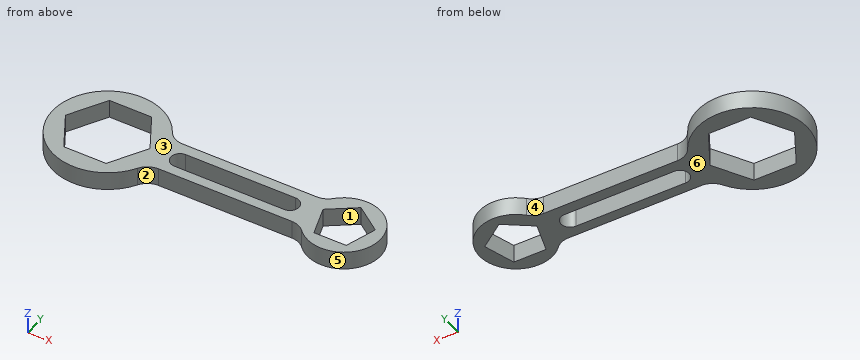
from build123d import *

# Parameters (mm, degrees)
BOSS_EXTRUDE1_DEPTH = 10


with BuildPart() as part:
    # Sketch1 → Boss-Extrude1 (new body)
    with BuildSketch(Plane.XY):
        with BuildLine():
            Line((34.148205858, 10.830267321), (107.410651623, 10.830267321))
            ThreePointArc((107.410651623, 10.830267321), (111.319985045, 11.626077395), (114.607101082, 13.886844881))
            ThreePointArc((114.607101082, 13.886844881), (148.999427872, -0.151277258), (114.398677604, -13.667530292))
            ThreePointArc((114.398677604, -13.667530292), (111.076857226, -11.326938473), (107.098016406, -10.501295438))
            Line((107.098016406, -10.501295438), (34.346715787, -10.501295438))
            ThreePointArc((34.346715787, -10.501295438), (29.409775368, -11.80493877), (25.76003684, -15.375971579))
            ThreePointArc((25.76003684, -15.375971579), (-29.999653993, -0.144084298), (25.611154394, 15.622700491))
            ThreePointArc((25.611154394, 15.622700491), (29.253089327, 12.110299767), (34.148205858, 10.830267321))
        make_face()
        Polygon((11.547005384, 20), (-11.547005384, 20), (-23.094010768, 0), (-11.547005384, -20), (11.547005384, -20), (23.094010768, 0), align=None, mode=Mode.SUBTRACT)
        Polygon((129, 15), (114.734152256, 4.635254916), (120.183221216, -12.135254916), (137.816778784, -12.135254916), (143.265847744, 4.635254916), align=None, mode=Mode.SUBTRACT)
        with BuildLine():
            Line((39.5, 5), (99.5, 5))
            ThreePointArc((99.5, 5), (104.5, 0), (99.5, -5))
            Line((99.5, -5), (39.5, -5))
            ThreePointArc((39.5, -5), (34.5, 0), (39.5, 5))
        make_face(mode=Mode.SUBTRACT)
    extrude(amount=BOSS_EXTRUDE1_DEPTH)


solid = part.part
The model under review builds one solid part; all positions refer to its coordinate system, in mm. Face numbers are marked on the shaded views. A direction names the side the tool comes from. Give positions to 0.01 mm unless a question says otherwise; leave off trailing zeros. Loops run counter-clockwise (first coordinate to the right, second up) from the corner with the lowest first, then second, coordinate; pieces in that order, holes last. Notation, with made-up numbers: (-22, 35.5) -> (24, 35.5) arc R27 ccw to (24, 70.5) -> close; hole circle Ø3 at (36.25, 23). An arc over 180 degrees is marked (long way). Put each result on its own line as item: value. Start each with the question number.
1. We need section A-A on x = 0. State the section outline as (y, z) points.
2. We need section C-C on y = 8. State the section outline as (x, z) points, then the cut area to 3 significant figures.
3. We need section B-B on z = 8. State the section outline as (x, y) points, then the cut area to 3 significant figures.
4. Wall thickness on probe 1 along Y at (x, z) = (76.5, 5.75); probe 2 along X at (y, z) = (-0.5, 9.25); probe 3 along X at (y, z) = (-16, 8): over which ranges is each line inside the solid? List them lowest first.
5. Clearance check with flat-ended pins moving along their axes: P1, Ø3, axis at y = 12.5, z = 6, coming from the +X side; P2, Ø5, axis at x = 85.5, z = 4.5, coming from the -Y side; P3, Ø1.5, axis at y = 12, z = 5, coming from the -X side. State where each tip first meets the part, or that it passes through.
6. We need section D-D on x = 92.5. State the section outline as (y, z) points, then the cut area to 3 significant figures.
7. Mouldability with a two-part tool opening along X and no side actions: class the marked faces 5 and 6 as released by +X, released by -X, zero draft, split by the parting line, or undercut.
8. For the marked faces 1, 2, 3 and 4, list the 3-axis set-ups (+Z, -Z, +X, -X, +Y, -Y) from which the entire face can be reached by the end or side of a thin tool; tool diameter is ignored.
Determined:
1. outline: (-30, 0) -> (-20, 0) -> (-20, 10) -> (-30, 10) -> close; (20, 0) -> (30, 0) -> (30, 10) -> (20, 10) -> close
2. outline: (-28.91, 0) -> (-18.48, 0) -> (-18.48, 10) -> (-28.91, 10) -> close; (18.48, 0) -> (119.37, 0) -> (119.37, 10) -> (18.48, 10) -> close; (138.63, 0) -> (147.33, 0) -> (147.33, 10) -> (138.63, 10) -> close
2. area: 1,200 mm^2
3. outline: (25.61, 15.62) arc R30 ccw (long way) to (25.76, -15.38) arc R10 cw to (34.35, -10.5) -> (107.1, -10.5) arc R10 cw to (114.4, -13.67) arc R20 ccw (long way) to (114.61, 13.89) arc R10 cw to (107.41, 10.83) -> (34.15, 10.83) arc R10 cw to start; hole (-23.09, 0) -> (-11.55, -20) -> (11.55, -20) -> (23.09, 0) -> (11.55, 20) -> (-11.55, 20) -> close; hole (39.5, -5) -> (99.5, -5) arc R5 ccw to (99.5, 5) -> (39.5, 5) arc R5 ccw to start; hole (114.73, 4.64) -> (120.18, -12.14) -> (137.82, -12.14) -> (143.27, 4.64) -> (129, 15) -> close
3. area: 3,220 mm^2
4. probe 1: -10.5 to -5, 5 to 10.83
4. probe 2: -30 to -22.81, 22.81 to 34.53, 104.47 to 116.4, 141.6 to 148.99
4. probe 3: -25.38 to -13.86, 13.86 to 25.38, 117 to 141
5. P1: x = 145.7
5. P2: y = -10.5
5. P3: x = -27.81
6. outline: (-10.5, 0) -> (-5, 0) -> (-5, 10) -> (-10.5, 10) -> close; (5, 0) -> (10.83, 0) -> (10.83, 10) -> (5, 10) -> close
6. area: 113 mm^2
7. face 5: undercut
7. face 6: zero draft
8. face 1: +Z, -Z
8. face 2: +Z, -Z, -Y
8. face 3: +Z, +X, -X, +Y, -Y
8. face 4: +Z, -Z, +Y
